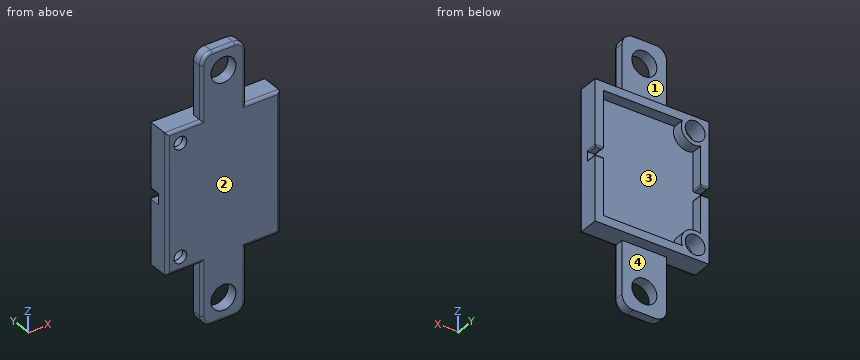
```python
from build123d import *

# Parameters (mm, degrees)
SKETCH2_W           = 20.5
SKETCH2_H           = 25
SKETCH2_R           = 1.15
BOSS_EXTRUDE1_DEPTH = 4
SKETCH3_OUTSIDE_W   = 29.016
SKETCH3_OUTSIDE_H   = 33.516
SKETCH3_OUTSIDE_W_2 = 20.5
SKETCH3_OUTSIDE_H_2 = 25
CUT_EXTRUDE1_DEPTH  = 2
SKETCH4_R           = 1.79
CUT_EXTRUDE2_DEPTH  = 2.92
DRAFT1_ANGLE        = 4
SKETCH5_W           = 8
SKETCH5_H           = 11.5
SKETCH5_R           = 2.2479
BOSS_EXTRUDE2_DEPTH = 2
FILLET1_R           = 2
FILLET2_R           = 0.5
SKETCH7_W           = 1.5
SKETCH7_H           = 2
CUT_EXTRUDE4_DEPTH  = 32.81587654
FILLET3_R           = 0.25


with BuildPart() as part:
    # Sketch2 → Boss-Extrude1 (new body)
    with BuildSketch(Plane(origin=(0, 0, 0), x_dir=(1, 0, 0), z_dir=(0, 1, 0))):
        Rectangle(SKETCH2_W, SKETCH2_H)
        with Locations(Location((-7.75, 10, 0), (0, 0, 270))):
            Circle(SKETCH2_R, mode=Mode.SUBTRACT)
        with Locations(Location((-7.75, -10, 0), (0, 0, 90))):
            Circle(SKETCH2_R, mode=Mode.SUBTRACT)
    extrude(amount=BOSS_EXTRUDE1_DEPTH)

    # Sketch3 outside → Cut-Extrude1 (cut)
    # profile 1 of 2: a face of its own
    with BuildSketch(Plane(origin=(0, 4, 0), x_dir=(1, 0, 0), z_dir=(0, 1, 0))):
        Rectangle(SKETCH3_OUTSIDE_W, SKETCH3_OUTSIDE_H)
        Rectangle(SKETCH3_OUTSIDE_W_2, SKETCH3_OUTSIDE_H_2, mode=Mode.SUBTRACT)
    # profile 2 of 2: a face of its own
    with BuildSketch(Plane(origin=(0, 4, 0), x_dir=(1, 0, 0), z_dir=(0, 1, 0))):
        with BuildLine():
            Line((-5.458712153, 11), (8.75, 11))
            Line((8.75, 11), (8.75, -11))
            Line((8.75, -11), (-5.458712153, -11))
            ThreePointArc((-5.458712153, -11), (-5.982233047, -8.232233047), (-8.75, -7.708712153))
            Line((-8.75, -7.708712153), (-8.75, 7.708712153))
            ThreePointArc((-8.75, 7.708712153), (-5.982233047, 8.232233047), (-5.458712153, 11))
        make_face()
    extrude(amount=-CUT_EXTRUDE1_DEPTH, mode=Mode.SUBTRACT)

    # Sketch4 → Cut-Extrude2 (cut)
    with BuildSketch(Plane(origin=(0, 4, 0), x_dir=(1, 0, 0), z_dir=(0, 1, 0))):
        with Locations(Location((-7.75, 10, 0), (0, 0, 270))):
            Circle(SKETCH4_R)
        with Locations(Location((-7.75, -10, 0), (0, 0, 90))):
            Circle(SKETCH4_R)
    extrude(amount=-CUT_EXTRUDE2_DEPTH, mode=Mode.SUBTRACT)

    # Draft1
    draft1_faces = [part.faces().sort_by_distance(p)[0] for p in [
        (-7.75, 2.54, 11.79),
        (-7.75, 2.54, -11.79),
    ]]
    draft(draft1_faces, Plane.ZX.offset(4), DRAFT1_ANGLE)

    # Sketch5 → Boss-Extrude2 (add)
    # profile 1 of 2: a face of its own
    with BuildSketch(Plane.XZ):
        with Locations((0, 18.25)):
            Rectangle(SKETCH5_W, SKETCH5_H)
        with Locations(Location((0, 20, 0), (0, 0, 270))):
            Circle(SKETCH5_R, mode=Mode.SUBTRACT)
    # profile 2 of 2: a face of its own
    with BuildSketch(Plane.XZ):
        with Locations((0, -18.25)):
            Rectangle(SKETCH5_W, SKETCH5_H)
        with Locations(Location((0, -20, 0), (0, 0, 90))):
            Circle(SKETCH5_R, mode=Mode.SUBTRACT)
    extrude(amount=-BOSS_EXTRUDE2_DEPTH)

    # Fillet1
    fillet1_edges = [part.edges().sort_by_distance(p)[0] for p in [
        (4, 1, 24),
        (-4, 1, 24),
        (4, 1, -24),
        (-4, 1, -24),
    ]]
    fillet(fillet1_edges, radius=FILLET1_R)

    # Fillet2
    fillet2_edges = [part.edges().sort_by_distance(p)[0] for p in [
        (7.125, 0, 12.5),
        (4, 0, 17.25),
        (-7.125, 0, -12.5),
        (-4, 0, -17.25),
        (0, 0, 24),
        (-4, 0, 17.25),
        (0, 0, -24),
        (4, 0, -17.25),
        (-3.414213562, 0, 23.414213562),
        (3.414213562, 0, 23.414213562),
        (3.414213562, 0, -23.414213562),
        (-3.414213562, 0, -23.414213562),
        (-7.125, 0, 12.5),
        (-10.25, 0, 0),
        (7.125, 0, -12.5),
        (10.25, 0, 0),
    ]]
    fillet(fillet2_edges, radius=FILLET2_R)

    # Sketch7 → Cut-Extrude4 (cut, through all)
    with BuildSketch(Plane.ZY.offset(10.25)):
        with Locations((0, 3)):
            Rectangle(SKETCH7_W, SKETCH7_H)
    extrude(amount=-CUT_EXTRUDE4_DEPTH, mode=Mode.SUBTRACT)

    # Fillet3
    fillet3_edges = [part.edges().sort_by_distance(p)[0] for p in [
        (9.5, 4, -0.75),
        (-9.5, 4, -0.75),
        (9.5, 4, 0.75),
        (8.75, 3, 0.75),
        (10.25, 3, 0.75),
        (-8.75, 3, 0.75),
        (-9.5, 4, 0.75),
        (8.75, 3, -0.75),
        (10.25, 3, -0.75),
        (-8.75, 3, -0.75),
        (-10.25, 3, 0.75),
        (-10.25, 3, -0.75),
    ]]
    fillet(fillet3_edges, radius=FILLET3_R)


solid = part.part
```
Model file for the job. Use its own axes, mm. Face numbers are marked on the shaded views. A direction names the side the tool comes from. Coordinates: 2 decimals unless noted, no trailing zeros. Write each loop counter-clockwise with the first axis right and the second up, starting at its lowest first coordinate (ties: lowest second). Pieces come first, ordered by that corner, then holes. Notation, with made-up numbers: (82.5, 77.25) - (101.5, 77.25) arc R25 cw to (101.5, 94.25) - close; hole circle Ø7 at (22.25, 85.25). An arc over 180 degrees is marked (long way). Use a Markdown table: item, result. Add a question column.
Item 1: Band-saw the part on C-C, the plane z = -20. Write the cut outline in (x, y).
Item 2: Band-saw the part on D-D, the plane x = -7.75. Write the cut outline in (y, z).
Item 3: Band-saw the part on A-A, the plane x = 0. Write the cut outline in (y, z).
Item 4: Drill centre lines: line 1 along Z through (x, y) = (-7.75, 0.4); line 2 along X through (y, z) = (2.4, 4.5); line 3 along X through (y, z) = (0.4, -10). Where is each one in solid material? Low to high.
Item 5: 3-axis set-ups, long thin cutter, end or side, ignore diameter. For the marked faces 1 and 2: which of +Z, -Z, +X, -X, +Y, -Y reach the whole face in a straight line?
Item 6: Band-saw the part on B-B, the plane z = 10. Write the cut outline in (x, y).
Item 7: Drop flat-ended pins along their axis: pin 1 (1.2 mm diameter, centred on y = 1, z = 18.5, fed in from +X); pin 2 (1.6 mm diameter, centred on x = 4, y = 3, fed in from +Z); pin 3 (0.5 mm diameter, centred on y = 1.5, z = 15.5, fed in from -X); pin 4 (2 mm diameter, centred on y = 3.5, z = 15, fed in from -X). Give the stop position or say it passes through.
Item 8: Two-plate mould, pull along Z, no slides. Class the marked faces 3 and 4: pulls with the +Z half, pulls with the -Z half, needs draft (parallel to the pull), parting line crosses it, or undercut.
A:
| question | item | result |
|---|---|---|
| 1 | outline | (-4, 0.5) arc R0.5 ccw to (-3.5, 0) - (-2.25, 0) - (-2.25, 2) - (-4, 2) - close; (2.25, 0) - (3.5, 0) arc R0.5 ccw to (4, 0.5) - (4, 2) - (2.25, 2) - close |
| 2 | outline | (0, -12) arc R0.5 ccw to (0.5, -12.5) - (4, -12.5) - (4, -11.79) - (1.08, -11.59) - (1.08, -11.15) - (0, -11.15) - close; (0, -8.85) - (1.08, -8.85) - (1.08, -8.41) - (4, -8.21) - (4, -7.5) - (2, -7.5) - (2, 7.5) - (4, 7.5) - (4, 8.21) - (1.08, 8.41) - (1.08, 8.85) - (0, 8.85) - close; (0, 11.15) - (1.08, 11.15) - (1.08, 11.59) - (4, 11.79) - (4, 12.5) - (0.5, 12.5) arc R0.5 ccw to (0, 12) - close |
| 3 | outline | (0, -23.5) arc R0.5 ccw to (0.5, -24) - (2, -24) - (2, -22.25) - (0, -22.25) - close; (0, -17.75) - (2, -17.75) - (2, -12.5) - (4, -12.5) - (4, -11) - (2, -11) - (2, 11) - (4, 11) - (4, 12.5) - (2, 12.5) - (2, 17.75) - (0, 17.75) - close; (0, 22.25) - (2, 22.25) - (2, 24) - (0.5, 24) arc R0.5 ccw to (0, 23.5) - close |
| 4 | line 1 | z = -12.49 to -11.15, -8.85 to 8.85, 11.15 to 12.49 |
| 4 | line 2 | x = -10.25 to -8.75, 8.75 to 10.25 |
| 4 | line 3 | x = -10.24 to -8.9, -6.6 to 10.24 |
| 5 | face 1 | +Z, +X, -X, +Y |
| 5 | face 2 | +Z, -Z, +X, -X, -Y |
| 6 | outline | (-10.25, 0.5) arc R0.5 ccw to (-9.75, 0) - (-8.9, 0) - (-8.9, 1.08) - (-9.34, 1.08) - (-9.54, 4) - (-10.25, 4) - close; (-6.6, 0) - (9.75, 0) arc R0.5 ccw to (10.25, 0.5) - (10.25, 4) - (8.75, 4) - (8.75, 2) - (-5.25, 2) - (-5.25, 4) - (-5.96, 4) - (-6.16, 1.08) - (-6.6, 1.08) - close |
| 7 | pin 1 | stops at x = 4 |
| 7 | pin 2 | stops at z = 12.5 |
| 7 | pin 3 | stops at x = -4 |
| 7 | pin 4 | passes through |
| 8 | face 3 | undercut |
| 8 | face 4 | needs draft |
